Autodesk Inventor part; units mm, degrees
ref_plane "РабПлоскость1" through (80, 0, 0) normal (1, 0, 0) x (0, 0, -1)
ref_plane "YZ Plane" through (0, 0, 0) normal (1, 0, 0) x (0, 1, 0)
ref_plane "XZ Plane" through (0, 0, 0) normal (0, 1, 0) x (-1, 0, 0)
sketch "Эскиз1" plane through (0, 0, 0) normal (1, 0, 0) x (0, 1, 0)
  circle A0 centre (0, 0) radius 7.5
  circle A1 centre (0, 0) radius 8.5
  dimension "d0" = 15
  dimension "d1" = 17
extrude "Выдавливание1" add sketch "Эскиз1" along normal blind 30
ref_plane "РабПлоскость1" through (80, 0, 0) normal (1, 0, 0) x (0, 0, -1)
sketch "Эскиз2" plane through (80, 0, 0) normal (1, 0, 0) x (0, 0, -1)
  circle A0 centre (0, 0) radius 8.5
  circle A1 centre (0, 0) radius 7.5
  dimension "d5" = 17
  dimension "d6" = 15
extrude "Выдавливание2" add sketch "Эскиз2" along normal blind 30
sketch "Эскиз3" plane through (0, 0, 0) normal (-1, 0, 0) x (0, 0, 1)
  circle A0 centre (0, 0) radius 7.5
  line L0 (-7.5, 0) -> (7.5, 0)
  circle A1 centre (0, 0) radius 8.5
  circle A2 centre (0, 0) radius 7.5
  circle A3 centre (0, 0) radius 8.5
  line L1 (8.2203, -2.1625) -> (12.2203, -2.1625)
  line L2 (8.2203, 2.1625) -> (12.2203, 2.1625)
  line L3 (12.2203, -2.1625) -> (12.2203, 2.1625)
  arc A4 (8.2203, -2.1625) -> (8.2203, 2.1625) centre (0, 0) ccw
  dimension "d9" = 4
extrude "Выдавливание3" add sketch "Эскиз3" against normal blind 110 contours A1 L2 L3 L1
sketch "Эскиз4" plane through (0, -2.1625, 12.2203) normal (0, 0, 1) x (1, 0, 0)
  line L0 (0, 4.325) -> (30, 4.325)
  line L1 (0, 0) -> (110, 0)
  line L2 (0, 4.325) -> (110, 4.325)
  line L3 (110, 4.325) -> (110, 0)
  line L4 (110, 0) -> (0, 0)
  line L5 (0, 0) -> (0, 4.325)
  line L6 (109, 1) -> (1, 1)
  line L7 (1, 1) -> (1, 3.325)
  line L8 (1, 3.325) -> (109, 3.325)
  line L9 (109, 3.325) -> (109, 1)
  line L10 (109, 1) -> (1, 3.325) construction
  line L11 (1, 1) -> (109, 3.325) construction
  line L12 (0, 4.325) -> (110, 4.325)
  line L13 (110, 0) -> (0, 0)
  line L14 (0, 0) -> (0, 4.325)
  line L15 (0, 4.325) -> (110, 4.325)
  line L16 (110, 4.325) -> (110, 0)
  line L17 (110, 0) -> (0, 4.325) construction
  line L18 (0, 0) -> (110, 4.325) construction
  point P0 (0, 2.1625)
  point P1 (55, 2.1625)
  point P2 (55, 2.1625)
  dimension "d12" = 108
  dimension "d13" = 2.325
extrude "Выдавливание4" add sketch "Эскиз4" along normal blind 180 contours L0 L2 L3 L1 L5 | L6 L7 L8 L9
sketch "Эскиз5" plane through (30, 2.1625, 8.2203) normal (0, 1, 0) x (1, 0, 0)
  line L0 (80, -184) -> (-30, -184)
  line L1 (25, -184) -> (25, -92)
  line L2 (-28, -2) -> (78, -2)
  line L3 (78, -2) -> (78, -182)
  line L4 (78, -182) -> (-28, -182)
  line L5 (-28, -182) -> (-28, -2)
  line L6 (-28, -2) -> (78, -182) construction
  line L7 (78, -2) -> (-28, -182) construction
  point P0 (-30, 8.2203)
  dimension "d16" = 92
  dimension "d17" = 106
  dimension "d18" = 180
extrude "Выдавливание5" cut sketch "Эскиз5" against normal blind 180
sketch "Эскиз6" plane through (108, 2.1625, 10.2203) normal (-1, 0, 0) x (0, 0, 1)
  line L0 (0, 0) -> (180, 0)
  line L1 (0, 0) -> (0, -1)
  line L2 (0, 0) -> (0, -4.325)
  line L3 (0, -1) -> (180, -1)
  line L4 (180, -1) -> (180, -3.325)
  line L5 (180, -3.325) -> (0, -3.325)
  line L6 (0, -3.325) -> (0, -1)
  point P0 (-10.2203, -2.1625)
  point P1 (0, -3.325)
  dimension "d21" = 1
  dimension "d22" = 2.325
extrude "Выдавливание6" cut sketch "Эскиз6" along normal blind 107 and the other way blind 1
properties part number "вращалка"
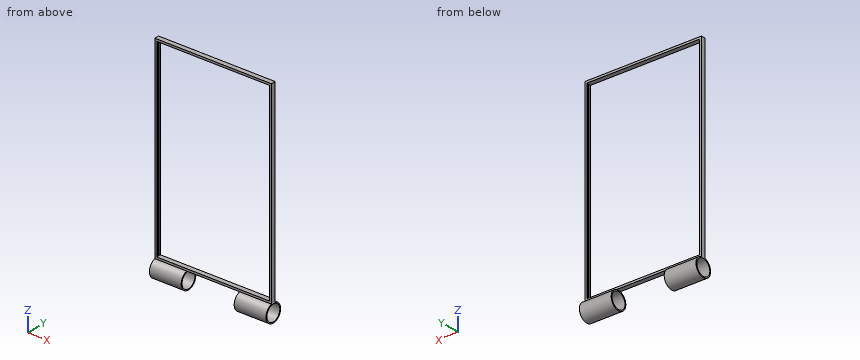
Work out the finished part from the listing and answer in its coordinate system (mm). Round coordinates to 2 decimals unless told otherwise and drop trailing zeros. Loops run counter-clockwise (first coordinate to the right, second up) from the corner with the lowest first, then second, coordinate; pieces in that order, holes last. Notation, with made-up numbers: (21, -28.75) - (53, -28.75) arc R11 cw to (53, -21.75) - close; hole circle Ø4 at (-1.75, -28.75). An arc over 180 degrees is marked (long way). One line per item, written item: value.
Q1. Find section A-A on z = 115. Give the vertices of the cut face in (x, y), and give its area (4 significant figures).
Check values:
outline: (0, -2.16) - (2, -2.16) - (2, -1.16) - (1, -1.16) - (1, 1.16) - (2, 1.16) - (2, 2.16) - (0, 2.16) - close; (108, -2.16) - (110, -2.16) - (110, 2.16) - (108, 2.16) - (108, 1.16) - (109, 1.16) - (109, -1.16) - (108, -1.16) - close
area: 12.65 mm2
Q2. Each of these flat-tipped pins is pushed along its axis until it touches: pin 1 Ø8 at (x, y) = (82.5, -5.5) entering from +Z; pin 2 Ø1.1 at (x, z) = (108.5, 57) entering from -Y; pin 3 Ø1.1 at (x, z) = (108.5, 89) entering from +Y; pin 4 Ø1 at (x, y) = (81.5, -6.5) entering from +Z. Where does it stop, or does it pass through?
Check values:
pin 1: z = 192.22
pin 2: y = -2.16
pin 3: y = 2.16
pin 4: z = 6.02
Q3. Straight lines are drawn through the part: probe 1 along Z at (x, y) = (19, 0); probe 2 along X at (y, z) = (-0.25, 43.5); probe 3 along Y at (x, z) = (97.5, 0). For each, find the intervals that lie inside material, in ascending order.
Check values:
probe 1: -8.5 to -7.5, 7.5 to 10.22, 190.22 to 192.22
probe 2: 0 to 1, 109 to 110
probe 3: -8.5 to -7.5, 7.5 to 8.5
Q4. Find section D-D on z = 0. Give the vertices of the cut face in (x, y).
Check values:
outline: (0, -8.5) - (30, -8.5) - (30, -7.5) - (0, -7.5) - close; (0, 7.5) - (30, 7.5) - (30, 8.5) - (0, 8.5) - close; (80, -8.5) - (110, -8.5) - (110, -7.5) - (80, -7.5) - close; (80, 7.5) - (110, 7.5) - (110, 8.5) - (80, 8.5) - close
Q5. Find section B-B on x = 36. Give the vertices of the cut face in (y, z).
Check values:
outline: (-2.16, 8.22) arc R8.5 cw to (2.16, 8.22) - (2.16, 10.22) - (-2.16, 10.22) - close; (-2.16, 190.22) - (2.16, 190.22) - (2.16, 192.22) - (-2.16, 192.22) - close
Q6. Find section C-C on y = -4. Give the vertices of the cut face in (x, z), and give its area (3 significant figures).
Check values:
outline: (0, -7.5) - (30, -7.5) - (30, -6.34) - (0, -6.34) - close; (0, 6.34) - (30, 6.34) - (30, 7.5) - (0, 7.5) - close; (80, -7.5) - (110, -7.5) - (110, -6.34) - (80, -6.34) - close; (80, 6.34) - (110, 6.34) - (110, 7.5) - (80, 7.5) - close
area: 139 mm2
